```python
from build123d import *

# Parameters (mm, degrees)
SKETCH_1_R      = 35.5
SKETCH_1_R_2    = 2
SKETCH_1_R_3    = 1.4
SKETCH_1_W      = 10
SKETCH_1_H      = 10
EXTRUDE_1_DEPTH = 4


with BuildPart() as part:
    # 草图1 → 凸台-拉伸1 (new body)
    with BuildSketch(Plane(origin=(0, 0, 0), x_dir=(1, 0, 0), z_dir=(0, 1, 0))):
        with BuildLine():
            Line((-77.023496261, 50), (77.023496261, 50))
            ThreePointArc((77.023496261, 50), (78.005849606, 49.902548511), (78.949910233, 49.613992762))
            ThreePointArc((78.949910233, 49.613992762), (112, 0), (78.949910233, -49.613992762))
            ThreePointArc((78.949910233, -49.613992762), (78.005849606, -49.902548511), (77.023496261, -50))
            Line((77.023496261, -50), (30, -50))
            Line((30, -50), (30, -40))
            Line((30, -40), (10, -40))
            Line((10, -40), (10, -50))
            Line((10, -50), (-10, -50))
            Line((-10, -50), (-10, -40))
            Line((-10, -40), (-30, -40))
            Line((-30, -40), (-30, -50))
            Line((-30, -50), (-77.023496261, -50))
            ThreePointArc((-77.023496261, -50), (-78.005849606, -49.902548511), (-78.949910233, -49.613992762))
            ThreePointArc((-78.949910233, -49.613992762), (-112, 0), (-78.949910233, 49.613992762))
            ThreePointArc((-78.949910233, 49.613992762), (-78.005849606, 49.902548511), (-77.023496261, 50))
        make_face()
        with Locations(Location((60, 0, 0), (0, 0, 270))):
            Circle(SKETCH_1_R, mode=Mode.SUBTRACT)
        with Locations(Location((60, 45, 0), (0, 0, 270))):
            Circle(SKETCH_1_R_2, mode=Mode.SUBTRACT)
        with Locations(Location((21.02885683, 22.5, 0), (0, 0, 270))):
            Circle(SKETCH_1_R_2, mode=Mode.SUBTRACT)
        with Locations(Location((21.02885683, -22.5, 0), (0, 0, 270))):
            Circle(SKETCH_1_R_2, mode=Mode.SUBTRACT)
        with Locations(Location((60, -45, 0), (0, 0, 270))):
            Circle(SKETCH_1_R_2, mode=Mode.SUBTRACT)
        with Locations(Location((98.97114317, -22.5, 0), (0, 0, 270))):
            Circle(SKETCH_1_R_2, mode=Mode.SUBTRACT)
        with Locations(Location((98.97114317, 22.5, 0), (0, 0, 270))):
            Circle(SKETCH_1_R_2, mode=Mode.SUBTRACT)
        with Locations(Location((-60, 0, 0), (0, 0, 270))):
            Circle(SKETCH_1_R, mode=Mode.SUBTRACT)
        with Locations(Location((-98.97114317, -22.5, 0), (0, 0, 270))):
            Circle(SKETCH_1_R_2, mode=Mode.SUBTRACT)
        with Locations(Location((-98.97114317, 22.5, 0), (0, 0, 270))):
            Circle(SKETCH_1_R_2, mode=Mode.SUBTRACT)
        with Locations(Location((-60, 45, 0), (0, 0, 270))):
            Circle(SKETCH_1_R_2, mode=Mode.SUBTRACT)
        with Locations(Location((-21.02885683, 22.5, 0), (0, 0, 270))):
            Circle(SKETCH_1_R_2, mode=Mode.SUBTRACT)
        with Locations(Location((-21.02885683, -22.5, 0), (0, 0, 270))):
            Circle(SKETCH_1_R_2, mode=Mode.SUBTRACT)
        with Locations(Location((-60, -45, 0), (0, 0, 270))):
            Circle(SKETCH_1_R_2, mode=Mode.SUBTRACT)
        with Locations(Location((-5, 45, 0), (0, 0, 270))):
            Circle(SKETCH_1_R_3, mode=Mode.SUBTRACT)
        with Locations(Location((5, 45, 0), (0, 0, 270))):
            Circle(SKETCH_1_R_3, mode=Mode.SUBTRACT)
        with Locations(Location((5, -45, 0), (0, 0, 270))):
            Circle(SKETCH_1_R_3, mode=Mode.SUBTRACT)
        with Locations(Location((-5, -45, 0), (0, 0, 270))):
            Circle(SKETCH_1_R_3, mode=Mode.SUBTRACT)
        with Locations(Location((-5, 0, 0), (0, 0, 270))):
            Circle(SKETCH_1_R_3, mode=Mode.SUBTRACT)
        with Locations(Location((5, 0, 0), (0, 0, 270))):
            Circle(SKETCH_1_R_3, mode=Mode.SUBTRACT)
        with Locations(Location((20, 45, 0), (0, 0, 270))):
            Circle(SKETCH_1_R_3, mode=Mode.SUBTRACT)
        with Locations(Location((30, 45, 0), (0, 0, 270))):
            Circle(SKETCH_1_R_3, mode=Mode.SUBTRACT)
        with Locations(Location((-30, 45, 0), (0, 0, 270))):
            Circle(SKETCH_1_R_3, mode=Mode.SUBTRACT)
        with Locations(Location((-20, 45, 0), (0, 0, 270))):
            Circle(SKETCH_1_R_3, mode=Mode.SUBTRACT)
        with Locations((-15, 35)):
            Rectangle(SKETCH_1_W, SKETCH_1_H, mode=Mode.SUBTRACT)
        with Locations((15, 35)):
            Rectangle(SKETCH_1_W, SKETCH_1_H, mode=Mode.SUBTRACT)
        with BuildLine():
            Line((-15.375343139, 28), (-4.5, 28))
            ThreePointArc((-4.5, 28), (-3.439339828, 27.560660172), (-3, 26.5))
            Line((-3, 26.5), (-3, 6.5))
            ThreePointArc((-3, 6.5), (-3.439339828, 5.439339828), (-4.5, 5))
            Line((-4.5, 5), (-8.508641502, 5))
            ThreePointArc((-8.508641502, 5), (-9.500661686, 5.374879583), (-9.996831054, 6.312138728))
            ThreePointArc((-9.996831054, 6.312138728), (-12.331318269, 16.366330744), (-16.665073106, 25.734104046))
            ThreePointArc((-16.665073106, 25.734104046), (-16.678961935, 27.242009457), (-15.375343139, 28))
        make_face(mode=Mode.SUBTRACT)
        with BuildLine():
            Line((15.375343139, 28), (4.5, 28))
            ThreePointArc((4.5, 28), (3.439339828, 27.560660172), (3, 26.5))
            Line((3, 26.5), (3, 6.5))
            ThreePointArc((3, 6.5), (3.439339828, 5.439339828), (4.5, 5))
            Line((4.5, 5), (8.508641502, 5))
            ThreePointArc((8.508641502, 5), (9.500661686, 5.374879583), (9.996831054, 6.312138728))
            ThreePointArc((9.996831054, 6.312138728), (12.331318269, 16.366330744), (16.665073106, 25.734104046))
            ThreePointArc((16.665073106, 25.734104046), (16.678961935, 27.242009457), (15.375343139, 28))
        make_face(mode=Mode.SUBTRACT)
        with BuildLine():
            Line((-3.5, -7.5), (-3.5, -32.5))
            ThreePointArc((-3.5, -32.5), (-3.939339828, -33.560660172), (-5, -34))
            Line((-5, -34), (-19.535694742, -34))
            ThreePointArc((-19.535694742, -34), (-20.888277371, -33.148475313), (-20.705183333, -31.560693642))
            ThreePointArc((-20.705183333, -31.560693642), (-13.794118714, -20.128997357), (-10.129021878, -7.283236994))
            ThreePointArc((-10.129021878, -7.283236994), (-9.625800595, -6.36528759), (-8.644766576, -6))
            Line((-8.644766576, -6), (-5, -6))
            ThreePointArc((-5, -6), (-3.939339828, -6.439339828), (-3.5, -7.5))
        make_face(mode=Mode.SUBTRACT)
        with BuildLine():
            Line((5, -6), (8.644766576, -6))
            ThreePointArc((8.644766576, -6), (9.625800595, -6.36528759), (10.129021878, -7.283236994))
            ThreePointArc((10.129021878, -7.283236994), (13.794118714, -20.128997357), (20.705183333, -31.560693642))
            ThreePointArc((20.705183333, -31.560693642), (20.888277371, -33.148475313), (19.535694742, -34))
            Line((19.535694742, -34), (5, -34))
            ThreePointArc((5, -34), (3.939339828, -33.560660172), (3.5, -32.5))
            Line((3.5, -32.5), (3.5, -7.5))
            ThreePointArc((3.5, -7.5), (3.939339828, -6.439339828), (5, -6))
        make_face(mode=Mode.SUBTRACT)
    extrude(amount=EXTRUDE_1_DEPTH)


solid = part.part
```
For this review, take the finished solid that the model builds, in its own axes (mm). A direction names the side the tool comes from. Give positions to 0.01 mm unless a question says otherwise; leave off trailing zeros. Write each loop counter-clockwise with the first axis right and the second up, starting at its lowest first coordinate (ties: lowest second). Pieces come first, ordered by that corner, then holes. Notation, with made-up numbers: M -31,-9.5 L 1,-9.5 A24 ccw 1,20.5 Z; hole C 31.5,-36 d2. An arc over 180 degrees is marked long. Answer as a JSON object with one key per item and string values. Group by question number.
Item 1: For pin 1 Ø1.2 at (y, z) = (1.5, -36.5) entering from +X; pin 2 Ø3 at (x, z) = (21.03, 22.5) entering from +Y; pin 3 Ø12 at (x, z) = (14.5, 35) entering from -Y; pin 4 Ø2 at (y, z) = (2, -19) entering from +X, all flat-tipped, find the tip position at first contact; note any pin that passes through.
Item 2: For probe 1 along X at (y, z) = (2.65, -19); probe 2 along X at (y, z) = (2.3, 1); probe 3 along Z at (x, y) = (79.5, 0.8), list the stretches that pass through material, from the lowest coordinate up. Write a range as [from, to].
Item 3: Consider section A-A on x = 60. Write out the cut boundary in (y, z).
Item 4: Consider section D-D on y = 1.6. Count the separate pieces of the cut face and the enclosed holes in it, plus the area to 3 significant figures.
Item 5: Consider section C-C on x = -72.5. Write out the cut boundary in (y, z).
Item 6: Consider section B-B on z = -13. Write out the cut boundary in (x, y), plus the area to 3 significant figures.
Item 7: Tool access review of faces 4 (the flat face through (-53, 2, 50)), 5 (the flat face through (-10, 2, -28)), 6 (the flat face through (-10, 2, 45)): name each direction out of +Z, -Z, +X, -X, +Y, -Y from which nothing blocks a thin tool from reaching the whole face with its end or side.
Item 8: Draft analysis for pull direction X (two halves, no side actions). For faces 1 (the cylindrical face through (111.993, 1.972, -0.885)), 2 (the flat face through (12, 2, 34)), 3 (the flat face through (2, 0, -1)), state which applies: +X half, -X half, draft (parallel to the pull), parting line (faces both ways), or undercut.
Check result:
{
 "1": {"pin 1": "stops at x = 98.26", "pin 2": "passes through", "pin 3": "stops at y = 0", "pin 4": "stops at x = 108.9"},
 "2": {"probe 1": "x = [-108.53, -89.99], [-30.01, -13.32], [-3, 3], [13.32, 30.01], [89.99, 108.53]", "probe 2": "x = [-111.99, -95.49], [-24.51, -5.98], [-4.02, 4.02], [5.98, 24.51], [95.49, 111.99]", "probe 3": "z = [-49.38, -29.66], [29.66, 49.38]"},
 "3": {"outline": "M 0,-50 L 4,-50 L 4,-47 L 0,-47 Z; M 0,-43 L 4,-43 L 4,-35.5 L 0,-35.5 Z; M 0,35.5 L 4,35.5 L 4,43 L 0,43 Z; M 0,47 L 4,47 L 4,50 L 0,50 Z"},
 "4": {"separate pieces": "1", "enclosed holes": "30", "area": "10,700 mm^2"},
 "5": {"outline": "M 0,-50 L 4,-50 L 4,-33.23 L 0,-33.23 Z; M 0,33.23 L 4,33.23 L 4,50 L 0,50 Z"},
 "6": {"outline": "M -110.4,0 L -93.03,0 L -93.03,4 L -110.4,4 Z; M -26.97,0 L -11.31,0 L -11.31,4 L -26.97,4 Z; M -3,0 L 3,0 L 3,4 L -3,4 Z; M 11.31,0 L 26.97,0 L 26.97,4 L 11.31,4 Z; M 93.03,0 L 110.4,0 L 110.4,4 L 93.03,4 Z", "area": "288 mm^2"},
 "7": {"face 4": "+Z, +X, -X, +Y, -Y", "face 5": "+Y, -Y", "face 6": "+Z, +Y, -Y"},
 "8": {"face 1": "+X half", "face 2": "undercut", "face 3": "draft"}
}
